Answer from the drawing. Dimensions are ordinates in mm from the lowest x, y and z of the part. A direction names the side the tool comes from. Round coordinates to 2 decimals unless told otherwise and drop trailing zeros. Write each loop counter-clockwise with the first axis right and the second up, starting at its lowest first coordinate (ties: lowest second). Pieces come first, ordered by that corner, then holes. Notation, with made-up numbers: (33.25, -21) - (57.25, -21) arc R24 cw to (57.25, -1) - close; hole circle Ø6 at (33.25, 72). An arc over 180 degrees is marked (long way). Use a Markdown table: item, result. Add a question column.
1) A cutting plane is placed at B-B (z = 16). Give the vertices of the cut face in (x, y) (3 decimals).
2) A cutting plane is placed at C-C (z = 52.5). Give the vertices of the cut face in (x, y) (3 decimals), then the cut area to 3 significant figures.
3) Determine the mould class of the marked faces 4 and 5 for opening direction Z: +Z half, -Z half, draft (parallel to the pull), parting line (faces both ways), or undercut.
4) Each of these flat-tipped pins is pushed along its axis until it touches: P1, Ø1, axis at y = 1.5, z = 11.5, coming from the -X side (3 decimals); P2, Ø1.5, axis at x = 26, y = 1.5, coming from the -Z side; P3, Ø2, axis at y = 1.5, z = 52.5, coming from the +X side (3 decimals); P4, Ø1, axis at x = 20, z = 62.5, coming from the -Y side. Where does it stop, or does it pass through?
5) A cutting plane is placed at A-A (x = 6). Give the vertices of the cut face in (y, z).
6) Find the intervals of material crossed by probe 1 along Z at (x, y) = (25.5, 1.5); probe 2 along Z at (x, y) = (3, 0.45); probe 3 along X at (y, z) = (2.25, 21) (3 decimals), in increasing order. Write a range as from..to.
7) A tool of negligible diameter and unlimited length cuts with its end or side. For the marked faces 1, 2 and 3, from which of +Z, -Z, +X, -X, +Y, -Y can it reach the whole face along a straight path? Write none if from no direction.
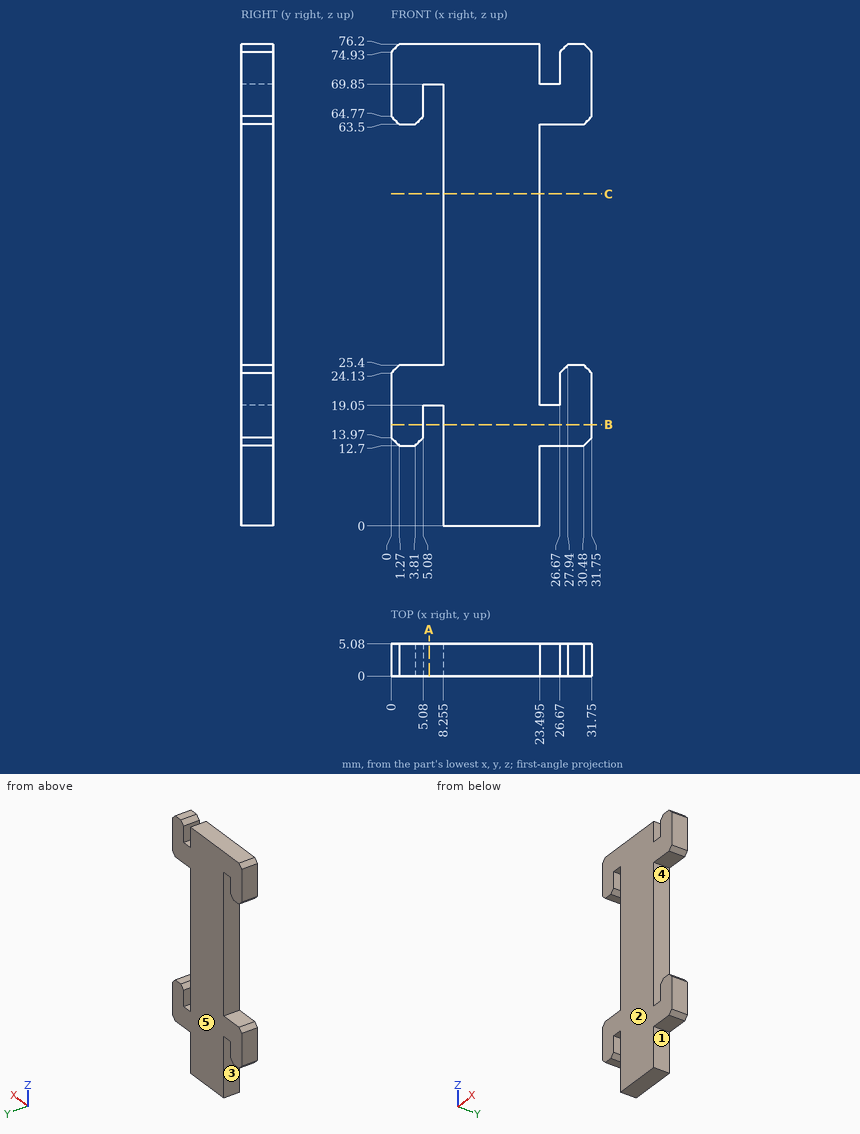
Entries:
| question | item | result |
|---|---|---|
| 1 | outline | (0, 0) - (5.08, 0) - (5.08, 5.08) - (0, 5.08) - close; (8.255, 0) - (31.75, 0) - (31.75, 5.08) - (8.255, 5.08) - close |
| 2 | outline | (8.255, 0) - (23.495, 0) - (23.495, 5.08) - (8.255, 5.08) - close |
| 2 | area | 77.4 mm² |
| 3 | face 4 | undercut |
| 3 | face 5 | draft |
| 4 | P1 | stops at x = 8.255 |
| 4 | P2 | stops at z = 12.7 |
| 4 | P3 | stops at x = 23.495 |
| 4 | P4 | stops at y = 0 |
| 5 | outline | (0, 19.05) - (5.08, 19.05) - (5.08, 25.4) - (0, 25.4) - close; (0, 69.85) - (5.08, 69.85) - (5.08, 76.2) - (0, 76.2) - close |
| 6 | probe 1 | z = 12.7..19.05, 63.5..69.85 |
| 6 | probe 2 | z = 12.7..25.4, 63.5..76.2 |
| 6 | probe 3 | x = 0..23.495, 26.67..31.75 |
| 7 | face 1 | -Z, +X, +Y, -Y |
| 7 | face 2 | +Z, -Z, +X, -X, -Y |
| 7 | face 3 | -Z, +Y, -Y |
